The figure shows three views and two pictorial views of one solid part (mm, origin at its lowest corner). Answer the questions. A direction names the side the tool comes from. Coordinates: 2 decimals unless noted, no trailing zeros. Order: outer loops, then holes, each group sorted by start corner. A loop starts at its lowest first (then second) coordinate and runs counter-clockwise, first axis right, second up. Notation, with made-up numbers: (-5, 79) -> (-1, 79) arc R21 cw to (-1, 99) -> close; hole circle Ø1 at (-24.5, 59.25). An arc over 180 degrees is marked (long way). Write item = value, one per line.
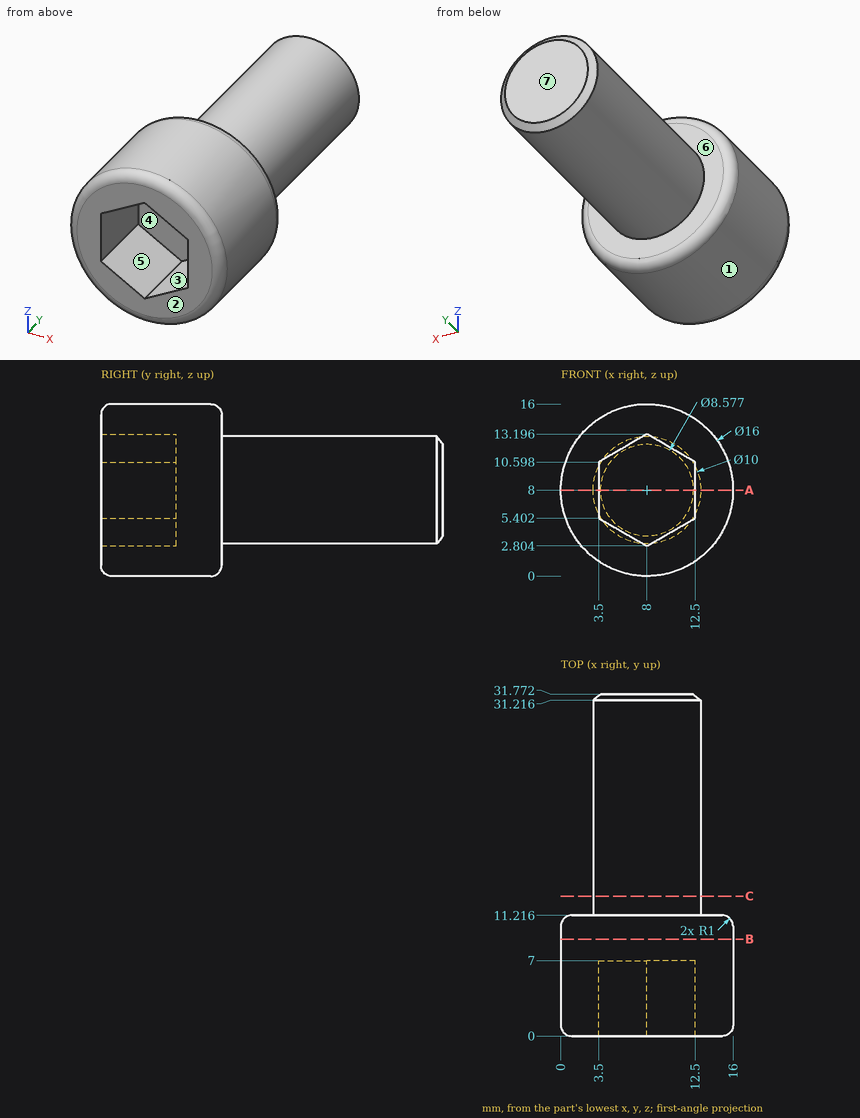
Q1. The mould has two halves that part along Z. Classify the marked faces 1, 2, 3 and 4: released by +Z, released by -Z, zero draft, split by the parting line, or undercut.
The answers:
face_1 = split by the parting line
face_2 = zero draft
face_3 = undercut
face_4 = undercut
Q2. Find the intervals of material crossed by line 1 along Y through (x, z) = (9.75, 8.5); line 2 along Y through (x, z) = (8.75, 14); line 3 along X through (y, z) = (6, 9.5), in increasing order.
The answers:
line_1 = 7 to 31.77
line_2 = 0 to 11.22
line_3 = 0.14 to 3.5, 12.5 to 15.86
Q3. Each of these flat-tipped pins is pushed along its axis until it touches: pin 1 Ø1 at (x, z) = (7.5, 9.5) entering from -Y; pin 2 Ø5 at (y, z) = (3.5, 4.5) entering from -X; pin 3 Ø1 at (x, z) = (13.5, 14) entering from -Y. Where does it stop, or does it pass through?
The answers:
pin_1 = 7
pin_2 = 0.06
pin_3 = 0.23
Q4. Section A-A, the plane z = 8 is taken. Give the vertices of the cut face in (x, y).
The answers:
outline = (0, 1) arc R1 ccw to (1, 0) -> (3.5, 0) -> (3.5, 7) -> (12.5, 7) -> (12.5, 0) -> (15, 0) arc R1 ccw to (16, 1) -> (16, 10.22) arc R1 ccw to (15, 11.22) -> (13, 11.22) -> (13, 31.22) -> (12.29, 31.77) -> (3.71, 31.77) -> (3, 31.22) -> (3, 11.22) -> (1, 11.22) arc R1 ccw to (0, 10.22) -> close
Q5. A tool of negligible diameter and unlimited length cuts with its end or side. For the marked faces 5, 6 and 7, from which of +Z, -Z, +X, -X, +Y, -Y can it reach the whole face along a straight path? Write none if from no direction.
The answers:
face_5 = -Y
face_6 = +Y
face_7 = +Z, -Z, +X, -X, +Y
Q6. Section B-B, the plane y = 9 is taken. Give the vertices of the cut face in (x, z), plus the area to 3 significant figures.
The answers:
outline = circle Ø16 at (8, 8)
area = 201 mm2
Q7. Section C-C, the plane y = 13 is taken. Give the vertices of the cut face in (x, z).
The answers:
outline = circle Ø10 at (8, 8)
